Part model, mm, in its own coordinate system. Face numbers are marked on the shaded views. Round coordinates to 2 decimals unless told otherwise and drop trailing zeros. Order: outer loops, then holes, each group sorted by start corner. A loop starts at its lowest first (then second) coordinate and runs counter-clockwise, first axis right, second up. Notation, with made-up numbers: (56, -25) -> (64, -25) arc R22 cw to (64, 9) -> close; hole circle Ø8 at (-18.5, 30.25). An arc over 180 degrees is marked (long way). Return JSON: item names as keys, results as strings. Group by question number.
from build123d import *

# Parameters (mm, degrees)
CHAMFER1_SIZE = 1.5
FILLET1_R     = 1


with BuildPart() as part:
    # Sketch1 → Revolve1 (revolve)
    with BuildSketch(Plane.XY, mode=Mode.PRIVATE) as revolve1_sk:
        Polygon((25, 4.05), (0, 4.05), (0, 10), (54, 10), (54, 6.5), (30, 6.5), (30, 2.775), (36, 2.775), (36, 0), (25, 0), align=None)
    revolve(revolve1_sk.sketch.rotate(Axis((0, 0, 0), (1, 0, 0)), 180), axis=Axis((0, 0, 0), (1, 0, 0)))

    # Chamfer1
    chamfer1_edges = [part.edges().sort_by_distance(p)[0] for p in [
        (0, 4.05, 0),
        (36, 2.775, 0),
        (54, 6.5, 0),
    ]]
    chamfer(chamfer1_edges, length=CHAMFER1_SIZE)

    # Fillet1
    fillet1_edges = [part.edges().sort_by_distance(p)[0] for p in [
        (54, 10, 0),
        (0, 10, 0),
    ]]
    fillet(fillet1_edges, radius=FILLET1_R)


solid = part.part
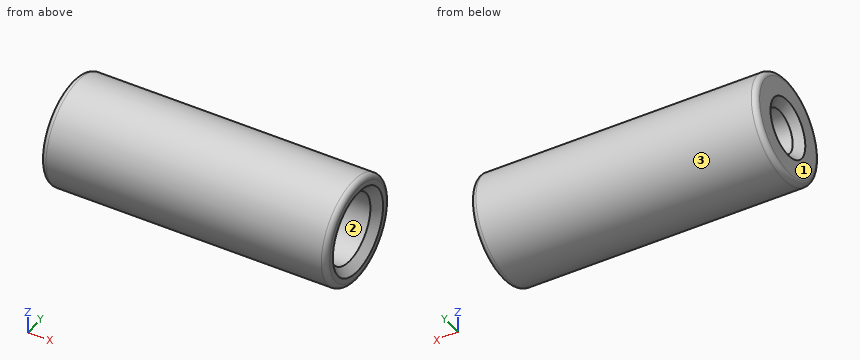
(1) Probe L1, parallel to Z at x = 47, y = 0; L2, parallel to Z at x = 15, y = 0; L3, parallel to Z at x = 35.25, y = 0 (3 decimals). List the from-to ranges inside material, lowest first. Write a range as [from, to].
(2) Mould opens along Z. For the marked faces 1, 2 and 3 say: pulls with the +Z half, pulls with the -Z half, needs draft (parallel to the pull), parting line crosses it, or undercut.
(3) Saw through at D-D, the plane x = 48. List the corners of the cut face in (y, z).
(4) Saw through at B-B, the plane z = 0. List the corners of the cut face in (x, y) (3 decimals), and give its area (3 significant figures).
(5) Saw through at A-A, the plane x = 8. List the corners of the cut face in (y, z), and give its area (3 significant figures).
(6) Pin check, flat tips, straight feed: P1, Ø10, axis at x = 12.5, z = -5.5, coming from the +Y side; P2, Ø3, axis at y = 0, z = 0, coming from the +X side; P3, Ø7.5, axis at y = 0, z = 0, coming from the -X side. Stop position of each tip, or through.
Results are:
{
 "1": {"L1": "z = [-10, -6.5], [6.5, 10]", "L2": "z = [-10, -4.05], [4.05, 10]", "L3": "z = [-10, -6.5], [-2.025, 2.025], [6.5, 10]"},
 "2": {"face 1": "needs draft", "face 2": "undercut", "face 3": "parting line crosses it"},
 "3": {"outline": "circle Ø20 at (0, 0); hole circle Ø13 at (0, 0)"},
 "4": {"outline": "(0, -9) arc R1 ccw to (1, -10) -> (53, -10) arc R1 ccw to (54, -9) -> (54, -8) -> (52.5, -6.5) -> (30, -6.5) -> (30, -2.775) -> (34.5, -2.775) -> (36, -1.275) -> (36, 1.275) -> (34.5, 2.775) -> (30, 2.775) -> (30, 6.5) -> (52.5, 6.5) -> (54, 8) -> (54, 9) arc R1 ccw to (53, 10) -> (1, 10) arc R1 ccw to (0, 9) -> (0, 5.55) -> (1.5, 4.05) -> (25, 4.05) -> (25, -4.05) -> (1.5, -4.05) -> (0, -5.55) -> close", "area": "591 mm^2"},
 "5": {"outline": "circle Ø20 at (0, 0); hole circle Ø8.1 at (0, 0)", "area": "263 mm^2"},
 "6": {"P1": "stops at y = 9.99", "P2": "stops at x = 36", "P3": "stops at x = 25"}
}
